Read the model definition and answer for the solid it produces. Units are mm, in the model's axes. A direction names the side the tool comes from. Round coordinates to 2 decimals unless told otherwise and drop trailing zeros. Loops run counter-clockwise (first coordinate to the right, second up) from the corner with the lowest first, then second, coordinate; pieces in that order, holes last. Notation, with made-up numbers: (25.25, 54.25) - (48.25, 54.25) arc R10 ccw to (48.25, 68.25) - close; hole circle Ø6 at (40.25, 13.25). An arc over 180 degrees is marked (long way). Answer as CSV lines item,"result".
```python
from build123d import *

# Parameters (mm, degrees)
ESQUISSE2_W                  = 6
ESQUISSE2_H                  = 7
ENL_V_MAT_EXTRU_1_DEPTH      = 3
R_P_TITION_CIRCULAIRE1_COUNT = 8
ESQUISSE3_R                  = 1.5
ENL_V_MAT_EXTRU_2_DEPTH      = 50.563091106


with BuildPart() as part:
    # Esquisse1 → Base-Révolution (revolve)
    with BuildSketch(Plane.XY, mode=Mode.PRIVATE) as base_r_volution_sk:
        Polygon((-24, 11), (0, 11), (0, 11.25), (1, 12.5), (6, 12.5), (6, 15.5), (-2, 15.5), (-2.5, 14.7), (-6, 14.7), (-6, 14.3), (-24, 14.3), align=None)
    revolve(base_r_volution_sk.sketch.rotate(Axis((0, 0, 0), (1, 0, 0)), 90), axis=Axis((0, 0, 0), (1, 0, 0)))

    # Esquisse2 → Enlèv. mat.-Extru.1 (cut)
    with BuildSketch(Plane(origin=(6, 0, 0), x_dir=(0, 0, -1), z_dir=(1, 0, 0))):
        with Locations((0, 13.5)):
            Rectangle(ESQUISSE2_W, ESQUISSE2_H)
    enl_v_mat_extru_1 = extrude(amount=-ENL_V_MAT_EXTRU_1_DEPTH, mode=Mode.SUBTRACT)

    # Répétition circulaire1: Enlèv. mat.-Extru.1 ×8 about axis
    r_p_tition_circulaire1_axis = Axis((0, 0, 0), (1, 0, 0))
    for i in range(1, R_P_TITION_CIRCULAIRE1_COUNT):
        add(enl_v_mat_extru_1.rotate(r_p_tition_circulaire1_axis, i * 360 / R_P_TITION_CIRCULAIRE1_COUNT), mode=Mode.SUBTRACT)

    # Esquisse3 → Enlèv. mat.-Extru.2 (cut, through all)
    with BuildSketch(Plane.XY.offset(25)):
        with Locations((-4, 0)):
            Circle(ESQUISSE3_R)
    extrude(amount=-ENL_V_MAT_EXTRU_2_DEPTH, mode=Mode.SUBTRACT)


solid = part.part
```
1) The mould has two halves that part along X. Classify faces 1 (the face through (-2.614, -0.575, -12.771)), 2 (the face through (5, -14, -3)), 3 (the face through (3, -14, 0)): pulls with the +X half, pulls with the -X half, needs draft (parallel to the pull), parting line crosses it, or undercut.
Entries:
face 1,"undercut"
face 2,"needs draft"
face 3,"pulls with the +X half"
2) Each of these flat-tipped pins is pushed along its axis until it touches: P1, Ø3, axis at x = 2.5, z = 2.5, coming from the +Y side; P2, Ø2, axis at x = -11, z = 3, coming from the +Y side; P3, Ø0.9, axis at x = 4, y = 13.5, coming from the +Z side. Where does it stop, or does it pass through?
Entries:
P1,"stops at y = 15.47"
P2,"stops at y = 14.16"
P3,"stops at z = 8.36"
3) A cutting plane is placed at B-B, the plane x = -12. Determine the outline of the cut face in (y, z), plus the area to 3 significant figures.
Entries:
outline,"circle Ø28.6 at (0, 0); hole circle Ø22 at (0, 0)"
area,"262 mm^2"
4) A tool of negligible diameter and unlimited length cuts with its end or side. For faces 4 (the face through (4.52, 11.77, -7.53)), 5 (the face through (3, 14, 0)), 6 (the face through (3, 10, 10)), 7 (the face through (5, 3, -14)), 8 (the face through (4.52, 11.77, 7.53)), from which of +Z, -Z, +X, -X, +Y, -Y can it reach the whole face along a straight path? Write none if from no direction.
Entries:
face 4,"-Z, +X"
face 5,"+X, +Y, -Y"
face 6,"+X"
face 7,"+Z, -Z, +X"
face 8,"+Z, +X"
5) A cutting plane is placed at A-A, the plane z = 0. Determine the outline of the cut face in (x, y), plus the area to 3 significant figures.
Entries:
outline,"(-24, -14.3) - (-6, -14.3) - (-6, -14.7) - (-2.5, -14.7) - (-2, -15.5) - (3, -15.5) - (3, -12.5) - (1, -12.5) - (0, -11.25) - (0, -11) - (-24, -11) - close; (-24, 11) - (0, 11) - (0, 11.25) - (1, 12.5) - (3, 12.5) - (3, 15.5) - (-2, 15.5) - (-2.5, 14.7) - (-6, 14.7) - (-6, 14.3) - (-24, 14.3) - close"
area,"186 mm^2"
6) Find the intervals of material crossed by line 1 (Y direction, x = 2, z = 0); line 2 (X direction, y = -13, z = -0.5); line 3 (Y direction, x = -21, z = 4), in increasing order.
Entries:
line 1,"y = -15.5 to -12.5, 12.5 to 15.5"
line 2,"x = -24 to 3"
line 3,"y = -13.73 to -10.25, 10.25 to 13.73"
